Geometry check sheet. Reference: the model listing, model coordinates, mm. A direction names the side the tool comes from. Round coordinates to 2 decimals unless told otherwise and drop trailing zeros. Order: outer loops, then holes, each group sorted by start corner. A loop starts at its lowest first (then second) coordinate and runs counter-clockwise, first axis right, second up.
(1) Gauge pin test, flat ends, axial feed: P1, Ø1.1, axis at x = -1.5, z = 1.5, coming from the -Y side; P2, Ø0.7, axis at x = 0, z = 1.5, coming from the -Y side; P3, Ø1.1, axis at y = -1, z = 1.5, coming from the -X side. Record the tip position at first contact, or that the pin passes through.
(2) Draft check along Y on faces 1 (the face through (0.5, 1.3, 1.5)), 2 (the face through (1, 2, 0)), 3 (the face through (0, -2, -3)). Enter one of: pulls with the +Y half, pulls with the -Y half, needs draft (parallel to the pull), parting line crosses it, or undercut.
(3) Thickness scan on L1, parallel to Y at x = 0.5, z = 0.75; L2, parallel to X at y = 1, z = -7; L3, parallel to Z at x = 1.5, y = -1.25. Record the ranges inside material, lowest first.
(4) Set-up check for faces 4 (the face through (0, -2, 1.4)), 5 (the face through (1.5, 0.5, 1.4)), 6 (the face through (0, 0, -7.3)): record each of +Z, -Z, +X, -X, +Y, -Y from which the full face is reachable in a straight line by a thin tool's end or side.
(5) Cross-section at A-A on z = -4.5. Enter the section's corners in (x, y), and give its area (3 significant figures).
from build123d import *

# Parameters (mm, degrees)
POCKET_DEPTH = 5


with BuildPart() as part:
    # Sketch → Revolution (revolve)
    with BuildSketch(Plane.XZ):
        with BuildLine():
            add(Edge.make_bspline(
                [(0, 2), (2.227338, 1.983256), (3.586166, 1.297371), (3.17254, 0), (2.834081, 0)],
                knots=[0, 0, 0, 0, 0.5, 1, 1, 1, 1], degree=3))
            Line((2.834081, 0), (2, 0))
            Line((2, 0), (2, -6.471573))
            Line((2, -6.471573), (1.171573, -7.3))
            Line((1.171573, -7.3), (0, -7.3))
            Line((0, -7.3), (0, 2))
        make_face()
    revolve(axis=Axis((0, 0, 0), (0, 0, 1)))

    # Sketch001 → Pocket (cut)
    with BuildSketch(Plane.XY.offset(1)):
        Polygon((-3.5, 0.5), (-0.5, 0.5), (-0.5, 2), (0.5, 2), (0.5, 0.5), (3.5, 0.5), (3.5, -0.5), (0.5, -0.5), (0.5, -2), (-0.5, -2), (-0.5, -0.5), (-3.5, -0.5), align=None)
    extrude(amount=POCKET_DEPTH, mode=Mode.SUBTRACT)


solid = part.part
Found:
1. P1: stops at y = -2.96
1. P2: stops at y = -3.14
1. P3: stops at x = -3.11
2. face 1: undercut
2. face 2: needs draft
2. face 3: parting line crosses it
3. L1: y = -3.2 to 3.2
3. L2: x = -1.08 to 1.08
3. L3: z = -6.52 to 1.84
4. face 4: +Z
4. face 5: +Z, +X, -X
4. face 6: -Z, +X, -X, +Y, -Y
5. outline: circle Ø4 at (0, 0)
5. area: 12.6 mm2
